from build123d import *

# Parameters (mm, degrees)
F0_W     = 90
F0_H     = 43.25
F1_DEPTH = 10
F2_R     = 12.5
F3_DEPTH = 15
F4_R     = 3.5
F5_DEPTH = 40


with BuildPart() as f1:
    # F0 (on Front) → F1 (new body, symmetric)
    with BuildSketch(Plane.XZ):
        Rectangle(F0_W, F0_H)
    extrude(amount=F1_DEPTH, both=True)

    # F2 (on Front) → F3 (cut, symmetric)
    with BuildSketch(Plane.XZ):
        with Locations((-30.016759, 22.333868)):
            Circle(F2_R)
        with Locations((29.983241, 22.534277)):
            Circle(F2_R)
    extrude(amount=F3_DEPTH, both=True, mode=Mode.SUBTRACT)

    # F4 (on Top) → F5 (cut, symmetric)
    with BuildSketch(Plane.XY):
        with Locations((-29.996643, 0)):
            Circle(F4_R)
        with Locations((29.950126, 0)):
            Circle(F4_R)
    extrude(amount=F5_DEPTH, both=True, mode=Mode.SUBTRACT)


solid = f1.part
Read the model definition and answer for the solid it produces. Units are mm, in the model's axes. Round coordinates to 2 decimals unless told otherwise and drop trailing zeros. Write each loop counter-clockwise with the first axis right and the second up, starting at its lowest first coordinate (ties: lowest second). Pieces come first, ordered by that corner, then holes.
1. The part is cut by section C-C, the plane y = 4.5. Determine the outline of the cut face in (x, z) (3 decimals), then the cut area to 3 significant figures.
2. The part is cut by section B-B, the plane y = -2.5. Determine the outline of the cut face in (x, z) (3 decimals).
3. Given pin 1 Ø9 at (x, y) = (29.95, 0) entering from -Z (3 decimals); pin 2 Ø12 at (x, y) = (35.5, -5) entering from +Z, each flat-ended and moving along its own axis, determine where each tip first touches the part or whether it passes through.
4. The part is cut by section D-D, the plane x = 32. Determine the outline of the cut face in (y, z) (3 decimals), then the cut area to 3 significant figures.
5. The part is cut by section A-A, the plane z = -15. Determine the outline of the cut face in (x, y).
6. Straight lines are drawn through the part: L1, parallel to X at y = 0, z = -1; L2, parallel to X at y = 0.25, z = 0.5; L3, parallel to Y at x = -27, z = -5. For each, find the intervals that lie inside material, in ascending order.
7. Determine the mould class of faces 1 (the face through (45, 0, 0)), 2 (the face through (-26.14, -0.14, 10.45)), 3 (the face through (-1, 0, -21.625)), 4 (the face through (-45, 0, 0)) for opening direction X: pulls with the +X half, pulls with the -X half, needs draft (parallel to the pull), parting line crosses it, or undercut.
Values:
1. outline: (-45, -21.625) - (45, -21.625) - (45, 21.625) - (42.45, 21.625) arc R12.5 cw to (17.516, 21.625) - (-17.537, 21.625) arc R12.5 cw to (-42.497, 21.625) - (-45, 21.625) - close
1. area: 3,440 mm2
2. outline: (-45, -21.625) - (-32.446, -21.625) - (-32.446, 10.072) arc R12.5 cw to (-42.497, 21.625) - (-45, 21.625) - close; (-27.547, -21.625) - (27.501, -21.625) - (27.501, 10.283) arc R12.5 cw to (17.516, 21.625) - (-17.537, 21.625) arc R12.5 cw to (-27.547, 10.08) - close; (32.4, -21.625) - (45, -21.625) - (45, 21.625) - (42.45, 21.625) arc R12.5 cw to (32.4, 10.27) - close
3. pin 1: stops at z = -21.625
3. pin 2: stops at z = 17.67
4. outline: (-10, -21.625) - (-2.837, -21.625) - (-2.837, 10.198) - (-10, 10.198) - close; (2.837, -21.625) - (10, -21.625) - (10, 10.198) - (2.837, 10.198) - close
4. area: 456 mm2
5. outline: (-45, -10) - (45, -10) - (45, 10) - (-45, 10) - close; hole circle Ø7 at (-30, 0); hole circle Ø7 at (29.95, 0)
6. L1: x = -45 to -33.5, -26.5 to 26.45, 33.45 to 45
6. L2: x = -45 to -33.49, -26.51 to 26.46, 33.44 to 45
6. L3: y = -10 to -1.81, 1.81 to 10
7. face 1: pulls with the +X half
7. face 2: undercut
7. face 3: needs draft
7. face 4: pulls with the -X half
